Read the model definition and answer for the solid it produces. Units are mm, in the model's axes. A direction names the side the tool comes from. Coordinates: 2 decimals unless noted, no trailing zeros. Write each loop counter-clockwise with the first axis right and the second up, starting at its lowest first coordinate (ties: lowest second). Pieces come first, ordered by that corner, then holes. Notation, with made-up numbers: M -7.5,38.25 L 32.5,38.25 A27 cw 32.5,66.25 Z; hole C 14,24 d6. An arc over 180 degrees is marked long. Write item = value, one per line.
from build123d import *

# Parameters (mm, degrees)
SKETCH1_R           = 12
SKETCH1_R_2         = 8.35
BOSS_EXTRUDE1_DEPTH = 1.5
SKETCH3_R           = 10.5
CUT_EXTRUDE1_DEPTH  = 0.1
SKETCH4_R           = 10.5
CUT_EXTRUDE2_DEPTH  = 0.1


with BuildPart() as part:
    # Sketch1 → Boss-Extrude1 (new body)
    with BuildSketch(Plane.XY):
        Circle(SKETCH1_R)
        Circle(SKETCH1_R_2, mode=Mode.SUBTRACT)
    extrude(amount=BOSS_EXTRUDE1_DEPTH)

    # Sketch3 → Cut-Extrude1 (cut)
    with BuildSketch(Plane.XY.offset(1.5)):
        Circle(SKETCH3_R)
    extrude(amount=-CUT_EXTRUDE1_DEPTH, mode=Mode.SUBTRACT)

    # Sketch4 → Cut-Extrude2 (cut)
    with BuildSketch(Plane(origin=(0, 0, 0), x_dir=(-1, 0, 0), z_dir=(0, 0, -1))):
        Circle(SKETCH4_R)
    extrude(amount=-CUT_EXTRUDE2_DEPTH, mode=Mode.SUBTRACT)


solid = part.part
Item 1: For a pull along X with two mould halves and no side action, classify faces 1 (the face through (7, -5, 0.1)), 2 (the face through (-11.99, 0.53, 0.74)), 3 (the face through (0, -11, 1.5)), 4 (the face through (7.964, 2.508, 0.741)) as released by +X, released by -X, zero draft, split by the parting line, or undercut.
Worked answers:
face_1 = undercut
face_2 = split by the parting line
face_3 = zero draft
face_4 = undercut
Item 2: Find section A-A (y = 0). Determine the outline of the cut face in (x, z).
Worked answers:
outline = M -12,0 L -10.5,0 L -10.5,0.1 L -8.35,0.1 L -8.35,1.4 L -10.5,1.4 L -10.5,1.5 L -12,1.5 Z; M 8.35,0.1 L 10.5,0.1 L 10.5,0 L 12,0 L 12,1.5 L 10.5,1.5 L 10.5,1.4 L 8.35,1.4 Z
Item 3: Which of the six approach directions +Z, -Z, +X, -X, +Y, -Y give full straight-line access (tool end or side, diameter ignored) to faces 5 (the face through (-7, -5, 1.4)), 6 (the face through (0, -11, 0))?
Worked answers:
face_5 = +Z
face_6 = -Z, +X, -X, +Y, -Y
Item 4: Consider line 1 along Z through (x, y) = (-5.75, -6.5); line 2 along Y through (x, z) = (0.75, 0.45); line 3 along X through (y, z) = (2.5, 1). Determine where each line is inside the solid, lowest interval first. Write a range as from..to.
Worked answers:
line_1 = 0.1..1.4
line_2 = -11.98..-8.32, 8.32..11.98
line_3 = -11.74..-7.97, 7.97..11.74
Item 5: Flat-ended cylindrical pins translate along their axes: pin 1 (10 mm diameter, centred on x = 0, y = 0, fed in from -Z); pin 2 (12 mm diameter, centred on x = 1, y = -4, fed in from +Z). Find the tip coordinate at first contact, or state that the pin passes through.
Worked answers:
pin_1 = through
pin_2 = 1.4
Item 6: Find section C-C (z = 0.45). Determine the outline of the cut face in (x, y), and give its area (3 significant figures).
Worked answers:
outline = C 0,0 d24; hole C 0,0 d16.7
area = 233 mm²
